Geometry: final body of the model. Coordinates: model frame, mm. Give positions to 0.01 mm unless a question says otherwise; leave off trailing zeros. One line per question, with ' | ' between items. Start each with the question number.
from build123d import *

# Parameters (mm, degrees)
SKETCH1_R             = 6.0625
SKETCH1_R_2           = 4.7625
BOSS_EXTRUDE1_DEPTH   = 3.175
SKETCH1_R_3           = 46.45
SKETCH1_R_4           = 44.45
BOSS_EXTRUDE1_2_DEPTH = 3.175
EXTRUDE_THIN2_START   = -3.175
EXTRUDE_THIN2_DEPTH   = 6.35
CIRPATTERN1_COUNT     = 8


# Read off the part's stored shape, not the designer's step: Extrude-Thin2
with BuildPart() as part:
    # Sketch1 → Boss-Extrude1 (new, symmetric)
    with BuildSketch(Plane(origin=(0, 0, 0), x_dir=(0, 0, -1), z_dir=(1, 0, 0))):
        Circle(SKETCH1_R)
        Circle(SKETCH1_R_2, mode=Mode.SUBTRACT)
    extrude(amount=BOSS_EXTRUDE1_DEPTH, both=True)



with BuildPart() as body_2:
    # Sketch1 → Boss-Extrude1 2 (new, symmetric)
    with BuildSketch(Plane(origin=(0, 0, 0), x_dir=(0, 0, -1), z_dir=(1, 0, 0))):
        Circle(SKETCH1_R_3)
        Circle(SKETCH1_R_4, mode=Mode.SUBTRACT)
    extrude(amount=BOSS_EXTRUDE1_2_DEPTH, both=True)


with BuildPart() as part_1:
    add(part.part)

    add(body_2.part)  # Extrude-Thin2 merges body 2
    # Extrude-Thin2 outline → Extrude-Thin2 (add)
    with BuildSketch(Plane(origin=(0, 0, 0), x_dir=(0, 0, -1), z_dir=(1, 0, 0)).offset(EXTRUDE_THIN2_START)):
        with BuildLine():
            add(Edge.make_bspline(
                [(-6.3355985, 43.996166784), (-6.255095923, 43.925032839), (-6.175963075, 43.852068198), (-5.548698351, 43.251204224), (-5.055604829, 42.640291134), (-4.116147204, 41.27108179), (-3.6714525, 40.51169877), (-2.385479272, 38.035518018), (-1.591781782, 36.118997617), (-0.134960901, 31.957605755), (0.525933851, 29.714211022), (1.670203871, 25.136721013), (2.153284246, 22.803242272), (2.890531028, 18.2847466), (3.145030649, 16.100931227), (3.311299949, 13.10122741), (3.330807031, 12.147155076), (3.286885537, 10.350080052), (3.224038366, 9.507507634), (2.992965499, 7.938587571), (2.827561189, 7.21225965), (2.459079192, 6.233276095), (2.328164202, 5.942334081), (2.170097204, 5.660793617)],
                knots=[0.116131233, 0.116131233, 0.116131233, 0.116131233, 0.125, 0.125, 0.1875, 0.1875, 0.25, 0.25, 0.375, 0.375, 0.5, 0.5, 0.625, 0.625, 0.75, 0.75, 0.8125, 0.8125, 0.875, 0.875, 0.9375, 0.9375, 0.965067589, 0.965067589, 0.965067589, 0.965067589], degree=3))
            ThreePointArc((-6.3355985, 43.996166784), (-8.165765838, 43.693509453), (-9.981711445, 43.31475426))
            add(Edge.make_bspline(
                [(-9.981711445, 43.31475426), (-3.408827872, 44.829448925), (4.490128061, 10.552628061), (0, 6.0625)],
                knots=[0, 0, 0, 0, 1, 1, 1, 1], degree=3))
            ThreePointArc((0, 6.0625), (1.103481977, 5.961227539), (2.170097204, 5.660793617))
        make_face()
    extrude_thin2 = extrude(amount=EXTRUDE_THIN2_DEPTH)

    # CirPattern1: Extrude-Thin2 ×8 about axis
    cirpattern1_axis = Axis((56.075510447, 0, 0), (-1, 0, 0))
    for i in range(1, CIRPATTERN1_COUNT):
        add(extrude_thin2.rotate(cirpattern1_axis, i * 360 / CIRPATTERN1_COUNT))


solid = part_1.part
(1) Contact query for flat-ended pins moving along their axis: P1, Ø2, axis at x = -0.5, z = 32.5, coming from the +Y side; P2, Ø2, axis at x = 1.5, y = -10, coming from the +Z side; P3, Ø11, axis at y = 0, z = 0, coming from the +X side (3 decimals); P4, Ø1, axis at x = 0.5, y = 4, coming from the -Z side. Output: stop coordinate, or through.
(2) Pull-direction query (Z, two-part tool) for faces 1 (the cylindrical face through (-0.044, -24.082, 37.361)), 2 (the flat face through (3.175, -3, 4)), 3 (the cylindrical face through (0.044, -45.345, 10.069)); classes: +Z half, -Z half, draft (parallel to the pull), parting line (faces both ways), or undercut.
(3) Material intervals for line 1 along Y through (x, z) = (-0.75, 33); line 2 along Z through (x, y) = (1, -15.5); line 3 along Y through (x, z) = (0.5, 27), sorted ascending. Write a range as from..to.
(4) Cut plane A-A, the plane x = -0.25. Give the number of separate pieces and of enclosed holes in the cut face, plus the area to 3 significant figures.
Results are:
1) P1: y = 34.14 | P2: z = 45.57 | P3: x = 3.175 | P4: z = -46.32
2) face 1: undercut | face 2: draft | face 3: parting line
3) line 1: -32.69..-29.78, -2.62..-0.51, 24.4..26.44, 29.78..32.69 | line 2: -43.79..-41.66, -15.06..-11.64, 1.15..3.16, 15.8..18.21, 41.66..43.79 | line 3: -37.8..-35.31, -0.86..1.2, 22.33..24.51, 35.31..37.8
4) separate pieces: 1 | enclosed holes: 9 | area: 1,260 mm2
